Geometry check sheet. Reference: the model listing, model coordinates, mm. Face numbers are marked on the shaded views. Round coordinates to 2 decimals unless told otherwise and drop trailing zeros. Order: outer loops, then holes, each group sorted by start corner. A loop starts at its lowest first (then second) coordinate and runs counter-clockwise, first axis right, second up.
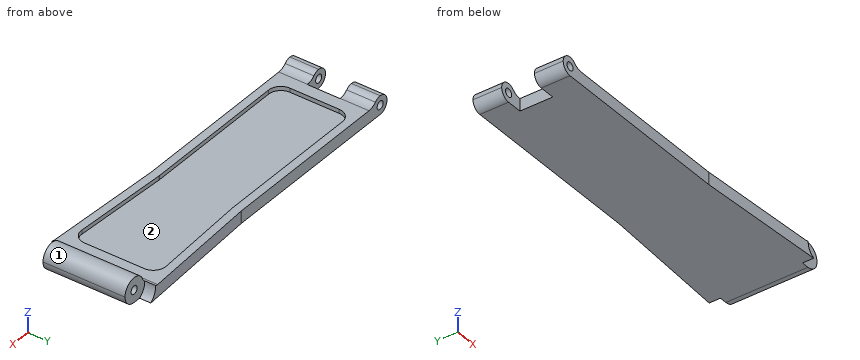
```python
from build123d import *

# Parameters (mm, degrees)
SALIENTE_EXTRUIR1_DEPTH = 3
CORTAR_EXTRUIR1_DEPTH   = 1
CROQUIS8_R              = 3
SALIENTE_EXTRUIR2_DEPTH = 12.5
REDONDEO1_R             = 3
CROQUIS9_R              = 3.5
CORTAR_EXTRUIR3_DEPTH   = 3
REDONDEO2_R             = 1.5
CROQUIS10_R             = 1
CORTAR_EXTRUIR4_DEPTH   = 15
REDONDEO3_R             = 3
SALIENTE_EXTRUIR3_DEPTH = 11
REDONDEO4_R             = 2.25
CROQUIS12_W             = 10
CROQUIS12_H             = 8
CORTAR_EXTRUIR5_DEPTH   = 22
CROQUIS13_R             = 1
CORTAR_EXTRUIR6_DEPTH   = 26
REDONDEO5_R             = 3
REDONDEO6_R             = 3


# Some blends are built 0.0001 mm under size
with BuildPart() as part:
    # Croquis1 → Saliente-Extruir1 (new body)
    with BuildSketch(Plane.XY):
        Polygon((0, 11), (-48, 11), (-48, -11), (0, -11), (37, -13), (37, 13), align=None)
    extrude(amount=SALIENTE_EXTRUIR1_DEPTH)

    # Croquis7 → Cortar-Extruir1 (cut)
    with BuildSketch(Plane.XY.offset(3)):
        Polygon((-39, 9), (-39, -9), (0.054014627, -9), (27, -10.45653975), (27, 10.45653975), (0.054014627, 9), align=None)
    extrude(amount=-CORTAR_EXTRUIR1_DEPTH, mode=Mode.SUBTRACT)

    # Croquis8 → Saliente-Extruir2 (add, symmetric)
    with BuildSketch(Plane(origin=(0, 0, 0), x_dir=(1, 0, 0), z_dir=(0, 1, 0))):
        with Locations((34, -3)):
            Circle(CROQUIS8_R)
    extrude(amount=SALIENTE_EXTRUIR2_DEPTH, both=True)

    # Redondeo1
    redondeo1_edges = [part.edges().sort_by_distance(p)[0] for p in [
        (37, 0, 0),
    ]]
    fillet(redondeo1_edges, radius=REDONDEO1_R - 0.0001)  # a hair under: the kernel refuses the full size

    # Croquis9 → Cortar-Extruir3 (cut)
    with BuildSketch(Plane(origin=(0, -13, 0), x_dir=(1, 0, 0), z_dir=(0, 1, 0))):
        with Locations((34, -3)):
            Circle(CROQUIS9_R)
    cortar_extruir3 = extrude(amount=CORTAR_EXTRUIR3_DEPTH, mode=Mode.SUBTRACT)

    # Simetría1: Cortar-Extruir3 across plane
    add(cortar_extruir3.mirror(Plane.ZX), mode=Mode.SUBTRACT)

    # Redondeo2
    redondeo2_edges = [part.edges().sort_by_distance(p)[0] for p in [
        (31, 0, 3),
    ]]
    fillet(redondeo2_edges, radius=REDONDEO2_R)

    # Croquis10 → Cortar-Extruir4 (cut, symmetric)
    with BuildSketch(Plane(origin=(0, 0, 0), x_dir=(1, 0, 0), z_dir=(0, 1, 0))):
        with Locations(Location((34, -3, 0), (0, 0, 270))):
            Circle(CROQUIS10_R)
    extrude(amount=CORTAR_EXTRUIR4_DEPTH, both=True, mode=Mode.SUBTRACT)

    # Redondeo3
    # the kernel refuses this fillet: 3 mm, written as the material it adds along each edge
    with BuildSketch(Plane(origin=(-39, -9, 3), x_dir=(0, 1, 0), z_dir=(0, 0, -1))) as redondeo3_piece_1:
        with BuildLine():
            CenterArc((REDONDEO3_R, REDONDEO3_R), REDONDEO3_R, 180, 90)
            Line((0, REDONDEO3_R), (0, 0))
            Line((0, 0), (REDONDEO3_R, 0))
        make_face()
    extrude(amount=1)
    with BuildSketch(Plane(origin=(-39, 9, 3), x_dir=(0, -1, 0), z_dir=(0, 0, -1))) as redondeo3_piece_2:
        with BuildLine():
            CenterArc((REDONDEO3_R, -REDONDEO3_R), REDONDEO3_R, 90, 90)
            Line((0, -REDONDEO3_R), (0, 0))
            Line((0, 0), (REDONDEO3_R, 0))
        make_face()
    extrude(amount=1)
    with BuildSketch(Plane(origin=(27, 10.45653975, 3), x_dir=(-0.9985422732775083, -0.053975258015000575, 0), z_dir=(0, 0, -1))) as redondeo3_piece_3:
        with BuildLine():
            CenterArc((REDONDEO3_R * 1.05551390885, -REDONDEO3_R), REDONDEO3_R, 90, 93.094058059)
            Line((REDONDEO3_R * 0.0569716355684, -REDONDEO3_R * 1.05397525801), (0, 0))
            Line((0, 0), (REDONDEO3_R * 1.05551390885, 0))
        make_face()
    extrude(amount=1)
    with BuildSketch(Plane(origin=(27, -10.45653975, 3), x_dir=(-0.9985422732775082, 0.053975258015002685, 0), z_dir=(0, 0, -1))) as redondeo3_piece_4:
        with BuildLine():
            CenterArc((REDONDEO3_R * 1.05551390885, REDONDEO3_R), REDONDEO3_R, 176.905941941, 93.094058059)
            Line((REDONDEO3_R * 0.0569716355684, REDONDEO3_R * 1.05397525802), (0, 0))
            Line((0, 0), (REDONDEO3_R * 1.05551390885, 0))
        make_face()
    extrude(amount=1)
    # the kernel refuses this fillet: 3 mm, written as the material it takes off along each edge
    with BuildSketch(Plane(origin=(0.054014627, 9, 3.202554852), x_dir=(-1, 0, 0), z_dir=(0, 0, -1))) as redondeo3_2_piece_1:
        with BuildLine():
            CenterArc((REDONDEO3_R * 0.0270073136489, REDONDEO3_R), REDONDEO3_R, 266.905941941, 3.094058059)
            Line((-REDONDEO3_R * 0.0269679443661, REDONDEO3_R * 0.00145772672249), (0, 0))
            Line((0, 0), (REDONDEO3_R * 0.0270073136489, 0))
        make_face()
    extrude(amount=1.202554852, mode=Mode.SUBTRACT)
    with BuildSketch(Plane(origin=(0.054014627, -9, 3.202554852), x_dir=(-1, 0, 0), z_dir=(0, 0, -1))) as redondeo3_2_piece_2:
        with BuildLine():
            CenterArc((REDONDEO3_R * 0.0270073136489, -REDONDEO3_R), REDONDEO3_R, 90, 3.094058059)
            Line((-REDONDEO3_R * 0.0269679443661, -REDONDEO3_R * 0.00145772672249), (0, 0))
            Line((0, 0), (REDONDEO3_R * 0.0270073136489, 0))
        make_face()
    extrude(amount=1.202554852, mode=Mode.SUBTRACT)

    # Croquis11 → Saliente-Extruir3 (add, symmetric)
    with BuildSketch(Plane(origin=(0, 0, 0), x_dir=(1, 0, 0), z_dir=(0, 1, 0))):
        with BuildLine():
            Line((-48, -4.5), (-45.75, -4.5))
            ThreePointArc((-45.75, -4.5), (-44.159009742, -3.840990258), (-43.5, -2.25))
            Line((-43.5, -2.25), (-43.5, 0))
            Line((-43.5, 0), (-48, 0))
            Line((-48, 0), (-48, -4.5))
        make_face()
    extrude(amount=SALIENTE_EXTRUIR3_DEPTH, both=True)

    # Redondeo4
    redondeo4_edges = [part.edges().sort_by_distance(p)[0] for p in [
        (-48, 0, 0),
        (-48, 0, 4.5),
    ]]
    fillet(redondeo4_edges, radius=REDONDEO4_R - 0.0001)  # a hair under: the kernel refuses the full size

    # Croquis12 → Cortar-Extruir5 (cut)
    with BuildSketch(Plane(origin=(0, 0, 0), x_dir=(-1, 0, 0), z_dir=(0, 0, -1))):
        with Locations((47, 0)):
            Rectangle(CROQUIS12_W, CROQUIS12_H)
    extrude(amount=-CORTAR_EXTRUIR5_DEPTH, mode=Mode.SUBTRACT)

    # Croquis13 → Cortar-Extruir6 (cut, symmetric)
    with BuildSketch(Plane(origin=(0, 0, 0), x_dir=(1, 0, 0), z_dir=(0, 1, 0))):
        with Locations(Location((-45.75, -2.25, 0), (0, 0, 180))):
            Circle(CROQUIS13_R)
    extrude(amount=CORTAR_EXTRUIR6_DEPTH, both=True, mode=Mode.SUBTRACT)

    # Redondeo5
    redondeo5_edges = [part.edges().sort_by_distance(p)[0] for p in [
        (-43.628679656, 7.5, 3),
        (-43.628679656, -7.5, 3),
    ]]
    fillet(redondeo5_edges, radius=REDONDEO5_R)

    # Redondeo6
    # the kernel refuses this fillet: 3 mm, written as the material it adds along each edge
    with BuildSketch(Plane(origin=(0, 11, 0), x_dir=(-1, 0, 0), z_dir=(0, 0, 1))) as redondeo6_piece_1:
        with BuildLine():
            CenterArc((REDONDEO6_R * 0.0270073136489, -REDONDEO6_R), REDONDEO6_R, 90, 3.094058059)
            Line((-REDONDEO6_R * 0.0269679443661, -REDONDEO6_R * 0.00145772672249), (0, 0))
            Line((0, 0), (REDONDEO6_R * 0.0270073136489, 0))
        make_face()
    extrude(amount=3)
    with BuildSketch(Plane(origin=(0, -11, 0), x_dir=(-1, 0, 0), z_dir=(0, 0, 1))) as redondeo6_piece_2:
        with BuildLine():
            CenterArc((REDONDEO6_R * 0.0270073136489, REDONDEO6_R), REDONDEO6_R, 266.905941941, 3.094058059)
            Line((-REDONDEO6_R * 0.0269679443661, REDONDEO6_R * 0.00145772672249), (0, 0))
            Line((0, 0), (REDONDEO6_R * 0.0270073136489, 0))
        make_face()
    extrude(amount=3)


solid = part.part
```
(1) Material ranges on line 1 (Z direction, x = -45.75, y = 8.25); line 2 (X direction, y = -1.5, z = 2.25); line 3 (Z direction, x = 13, y = 5.75), recorded low to high.
Returned:
line 1: z = 0 to 1.25, 3.25 to 4.5
line 2: x = -42 to -39, 27 to 33.34, 34.66 to 36.9
line 3: z = 0 to 2
(2) Depth check by flat-ended pin: P1, Ø1.3, axis at x = -46.5, z = 2.5, coming from the -Y side; P2, Ø10.5, axis at x = 5, y = -1, coming from the +Z side; P3, Ø3, axis at x = -22.5, z = 3.5, coming from the +Y side. Enter the tip coordinate at first touch or a pass-through.
Returned:
P1: stops at y = -11
P2: stops at z = 2
P3: stops at y = 11
(3) Draft check along Y on the marked faces 1 and 2. Enter one of: released by +Y, released by -Y, zero draft, split by the parting line, or undercut.
Returned:
face 1: zero draft
face 2: undercut
(4) Sectioned sample at B-B, the plane x = 18. Record the cut outline in (y, z), and give its area (3 significant figures).
Returned:
outline: (-11.97, 0) - (11.97, 0) - (11.97, 3) - (9.97, 3) - (9.97, 2) - (-9.97, 2) - (-9.97, 3) - (-11.97, 3) - close
area: 51.9 mm2
